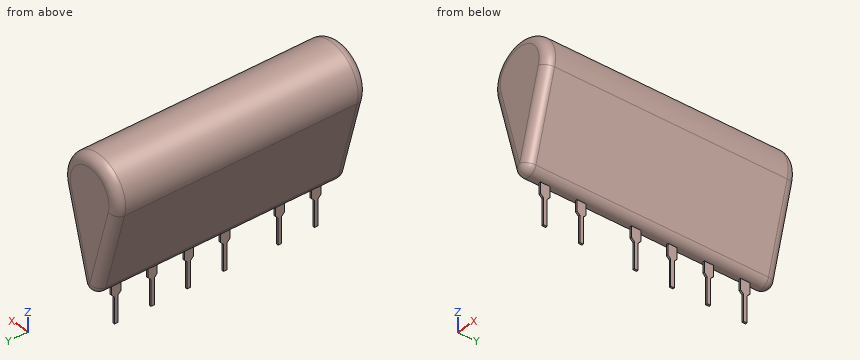
```python
from build123d import *

# Parameters (mm, degrees)
BOSS_EXTRUDE1_DEPTH = 17.5
FILLET1_R           = 1.27
SKETCH2_W           = 0.25
SKETCH2_H           = 1.3
BOSS_EXTRUDE2_DEPTH = 6
CUT_EXTRUDE1_REACH  = 28.615
LPATTERN1_COUNT     = 4
LPATTERN1_PITCH     = 5.08
SKETCH4_W           = 0.25
SKETCH4_H           = 1.3
BOSS_EXTRUDE3_DEPTH = 6
CUT_EXTRUDE2_REACH  = 28.615
LPATTERN3_COUNT     = 2
LPATTERN3_PITCH     = 5.08


with BuildPart() as part:
    # Sketch1 → Boss-Extrude1 (new, symmetric)
    with BuildSketch(Plane(origin=(0, 0, 0), x_dir=(1, 0, 0), z_dir=(0, 1, 0))):
        with BuildLine():
            Line((-1.223083707, -2.427996716), (-4.381914067, -13.724712644))
            ThreePointArc((-4.381914067, -13.724712644), (0, -19.5), (4.381914067, -13.724712644))
            Line((4.381914067, -13.724712644), (1.223083707, -2.427996716))
            ThreePointArc((1.223083707, -2.427996716), (0, -1.5), (-1.223083707, -2.427996716))
        make_face()
    extrude(amount=BOSS_EXTRUDE1_DEPTH, both=True)

    # Fillet1
    fillet1_edges = [part.edges().sort_by_distance(p)[0] for p in [
        (0, 17.5, 19.5),
        (2.802498887, 17.5, 8.07635468),
        (0, 17.5, 1.5),
        (2.802498887, -17.5, 8.07635468),
        (0, -17.5, 19.5),
        (-2.802498887, -17.5, 8.07635468),
        (0, -17.5, 1.5),
        (-2.802498887, 17.5, 8.07635468),
    ]]
    fillet(fillet1_edges, radius=FILLET1_R)

    # Sketch2 → Boss-Extrude2 (add)
    with BuildSketch(Plane.XY.offset(2)):
        with Locations((0, 13.9)):
            Rectangle(SKETCH2_W, SKETCH2_H)
    boss_extrude2 = extrude(amount=-BOSS_EXTRUDE2_DEPTH)

    # Sketch3 → Cut-Extrude1 (cut, up to next)
    with BuildSketch(Plane(origin=(0.125, 0, 0), x_dir=(0, 0, -1), z_dir=(1, 0, 0)), mode=Mode.PRIVATE) as cut_extrude1_sk1:
        Polygon((4, 14.150000008), (0.399999992, 14.150000008), (0, 14.55), (4, 14.55), align=None)
    cut_extrude1_tool1 = extrude(cut_extrude1_sk1.sketch, amount=-CUT_EXTRUDE1_REACH, mode=Mode.PRIVATE) & part.part
    # Sketch3 → Cut-Extrude1 (cut, up to next)
    with BuildSketch(Plane(origin=(0.125, 0, 0), x_dir=(0, 0, -1), z_dir=(1, 0, 0)), mode=Mode.PRIVATE) as cut_extrude1_sk2:
        Polygon((4, 13.25), (4, 13.649999992), (0.399999992, 13.649999992), (0, 13.25), align=None)
    cut_extrude1_tool2 = extrude(cut_extrude1_sk2.sketch, amount=-CUT_EXTRUDE1_REACH, mode=Mode.PRIVATE) & part.part
    cut_extrude1_1 = cut_extrude1_tool1.solids().sort_by_distance((0.125, 14.353509, -2.098246))[0]
    add(cut_extrude1_1, mode=Mode.SUBTRACT)
    cut_extrude1_2 = cut_extrude1_tool2.solids().sort_by_distance((0.125, 13.446491, -2.098246))[0]
    add(cut_extrude1_2, mode=Mode.SUBTRACT)
    cut_extrude1 = cut_extrude1_1 + cut_extrude1_2  # Cut-Extrude1 as one shape, for the pattern or mirror that repeats it

    # LPattern1: Boss-Extrude2, Cut-Extrude1 ×4
    with Locations(*[(0, -i * LPATTERN1_PITCH, 0) for i in range(1, LPATTERN1_COUNT)]):
        add(boss_extrude2)
        add(cut_extrude1, mode=Mode.SUBTRACT)

    # Sketch4 → Boss-Extrude3 (add)
    with BuildSketch(Plane.XY.offset(2)):
        with Locations((0, -8.96)):
            Rectangle(SKETCH4_W, SKETCH4_H)
    boss_extrude3 = extrude(amount=-BOSS_EXTRUDE3_DEPTH)

    # Sketch5 → Cut-Extrude2 (cut, up to next)
    with BuildSketch(Plane(origin=(0.125, 0, 0), x_dir=(0, 0, -1), z_dir=(1, 0, 0)), mode=Mode.PRIVATE) as cut_extrude2_sk1:
        Polygon((4, -8.709999992), (0.399999992, -8.709999992), (0, -8.31), (4, -8.31), align=None)
    cut_extrude2_tool1 = extrude(cut_extrude2_sk1.sketch, amount=-CUT_EXTRUDE2_REACH, mode=Mode.PRIVATE) & part.part
    # Sketch5 → Cut-Extrude2 (cut, up to next)
    with BuildSketch(Plane(origin=(0.125, 0, 0), x_dir=(0, 0, -1), z_dir=(1, 0, 0)), mode=Mode.PRIVATE) as cut_extrude2_sk2:
        Polygon((4, -9.61), (4, -9.210000008), (0.399999992, -9.210000008), (0, -9.61), align=None)
    cut_extrude2_tool2 = extrude(cut_extrude2_sk2.sketch, amount=-CUT_EXTRUDE2_REACH, mode=Mode.PRIVATE) & part.part
    cut_extrude2_1 = cut_extrude2_tool1.solids().sort_by_distance((0.125, -8.506491, -2.098246))[0]
    add(cut_extrude2_1, mode=Mode.SUBTRACT)
    cut_extrude2_2 = cut_extrude2_tool2.solids().sort_by_distance((0.125, -9.413509, -2.098246))[0]
    add(cut_extrude2_2, mode=Mode.SUBTRACT)
    cut_extrude2 = cut_extrude2_1 + cut_extrude2_2  # Cut-Extrude2 as one shape, for the pattern or mirror that repeats it

    # LPattern3: Boss-Extrude3, Cut-Extrude2 ×2
    with Locations(*[(0, -i * LPATTERN3_PITCH, 0) for i in range(1, LPATTERN3_COUNT)]):
        add(boss_extrude3)
        add(cut_extrude2, mode=Mode.SUBTRACT)


solid = part.part
```
Here's how the part is built. I have some questions about the finished solid (model axes, mm). Round coordinates to 2 decimals unless told otherwise and drop trailing zeros. Write each loop counter-clockwise with the first axis right and the second up, starting at its lowest first coordinate (ties: lowest second). Pieces come first, ordered by that corner, then holes.
Q1. Will these pins go through, and if not, where does the flat tip stop? P1, Ø0.7, axis at y = 14, z = -2, coming from the -X side (3 decimals); P2, Ø1, axis at y = 9, z = -1, coming from the +X side (3 decimals); P3, Ø3, axis at x = 3, z = 11, coming from the -Y side; P4, Ø2, axis at x = 2.5, y = -8, coming from the +Z side.
Q2. If we section it at A-A on y = 2: Write out the boundary of the cut face in (x, z).
Q3. Please list where these lines run through material, in increasing order: probe 1 along Y at (x, z) = (0, 1.25); probe 2 along Y at (x, z) = (0.75, 3.25); probe 3 along X at (y, z) = (4.5, 16.75).
Answer below:
1. P1: stops at x = -0.125
1. P2: stops at x = 0.125
1. P3: stops at y = -17.5
1. P4: stops at z = 19.25
2. outline: (-4.38, 13.72) - (-1.22, 2.43) arc R1.27 ccw to (1.22, 2.43) - (4.38, 13.72) arc R4.55 ccw (long way) to start
3. probe 1: y = -14.69 to -13.39, -9.61 to -8.31, -1.99 to -0.69, 3.09 to 4.39, 8.17 to 9.47, 13.25 to 14.55
3. probe 2: y = -17.35 to 17.35
3. probe 3: x = -4.18 to 4.18
